from build123d import *

# Parameters (mm, degrees)
SKETCH1_W           = 381
SKETCH1_H           = 508
BOSS_EXTRUDE1_DEPTH = 4.7625
SKETCH2_R           = 14.3383
SKETCH2_R_2         = 2.54
CUT_EXTRUDE1_DEPTH  = 4.7625
SKETCH3_R           = 2.413
CUT_EXTRUDE2_DEPTH  = 4.7625
FILLET1_R           = 2.54


with BuildPart() as part:
    # Sketch1 → Boss-Extrude1 (new body)
    with BuildSketch(Plane(origin=(0, 0, 0), x_dir=(1, 0, 0), z_dir=(0, 1, 0))):
        Rectangle(SKETCH1_W, SKETCH1_H)
    extrude(amount=BOSS_EXTRUDE1_DEPTH)

    # Sketch2 → Cut-Extrude1 (cut)
    with BuildSketch(Plane(origin=(0, 4.7625, 0), x_dir=(1, 0, 0), z_dir=(0, 1, 0))):
        with Locations(Location((-139.7, 228.6, 0), (0, 0, 270))):
            Circle(SKETCH2_R)
        with Locations(Location((-157.660512242, 246.560512242, 0), (0, 0, 270))):
            Circle(SKETCH2_R_2)
        with Locations(Location((-121.739487758, 246.560512242, 0), (0, 0, 270))):
            Circle(SKETCH2_R_2)
        with Locations(Location((-121.739487758, 210.639487758, 0), (0, 0, 270))):
            Circle(SKETCH2_R_2)
        with Locations(Location((-157.660512242, 210.639487758, 0), (0, 0, 270))):
            Circle(SKETCH2_R_2)
        with Locations(Location((-139.7, 177.8, 0), (0, 0, 270))):
            Circle(SKETCH2_R)
        with Locations(Location((-121.739487758, 195.760512242, 0), (0, 0, 270))):
            Circle(SKETCH2_R_2)
        with Locations(Location((-157.660512242, 195.760512242, 0), (0, 0, 270))):
            Circle(SKETCH2_R_2)
        with Locations(Location((-157.660512242, 159.839487758, 0), (0, 0, 270))):
            Circle(SKETCH2_R_2)
        with Locations(Location((-121.739487758, 159.839487758, 0), (0, 0, 270))):
            Circle(SKETCH2_R_2)
        with Locations(Location((-139.7, 127, 0), (0, 0, 270))):
            Circle(SKETCH2_R)
        with Locations(Location((-121.739487758, 144.960512242, 0), (0, 0, 270))):
            Circle(SKETCH2_R_2)
        with Locations(Location((-157.660512242, 144.960512242, 0), (0, 0, 270))):
            Circle(SKETCH2_R_2)
        with Locations(Location((-157.660512242, 109.039487758, 0), (0, 0, 270))):
            Circle(SKETCH2_R_2)
        with Locations(Location((-121.739487758, 109.039487758, 0), (0, 0, 270))):
            Circle(SKETCH2_R_2)
        with Locations(Location((-139.7, 76.2, 0), (0, 0, 270))):
            Circle(SKETCH2_R)
        with Locations(Location((-121.739487758, 94.160512242, 0), (0, 0, 270))):
            Circle(SKETCH2_R_2)
        with Locations(Location((-157.660512242, 94.160512242, 0), (0, 0, 270))):
            Circle(SKETCH2_R_2)
        with Locations(Location((-157.660512242, 58.239487758, 0), (0, 0, 270))):
            Circle(SKETCH2_R_2)
        with Locations(Location((-121.739487758, 58.239487758, 0), (0, 0, 270))):
            Circle(SKETCH2_R_2)
    extrude(amount=-CUT_EXTRUDE1_DEPTH, mode=Mode.SUBTRACT)

    # Sketch3 → Cut-Extrude2 (cut)
    with BuildSketch(Plane(origin=(0, 4.7625, 0), x_dir=(1, 0, 0), z_dir=(0, 1, 0))):
        with Locations(Location((165.1, 228.6, 0), (0, 0, 270))):
            Circle(SKETCH3_R)
        with Locations(Location((165.1, 177.8, 0), (0, 0, 270))):
            Circle(SKETCH3_R)
        with Locations(Location((165.1, 127, 0), (0, 0, 270))):
            Circle(SKETCH3_R)
        with Locations(Location((165.1, 76.2, 0), (0, 0, 270))):
            Circle(SKETCH3_R)
        with Locations(Location((165.1, 25.4, 0), (0, 0, 270))):
            Circle(SKETCH3_R)
        with Locations(Location((165.1, -25.4, 0), (0, 0, 270))):
            Circle(SKETCH3_R)
        with Locations(Location((165.1, -76.2, 0), (0, 0, 270))):
            Circle(SKETCH3_R)
        with Locations(Location((165.1, -127, 0), (0, 0, 270))):
            Circle(SKETCH3_R)
        with Locations(Location((165.1, -177.8, 0), (0, 0, 270))):
            Circle(SKETCH3_R)
        with Locations(Location((165.1, -228.6, 0), (0, 0, 270))):
            Circle(SKETCH3_R)
        with Locations(Location((139.7, 177.8, 0), (0, 0, 270))):
            Circle(SKETCH3_R)
        with Locations(Location((139.7, 127, 0), (0, 0, 270))):
            Circle(SKETCH3_R)
        with Locations(Location((139.7, 76.2, 0), (0, 0, 270))):
            Circle(SKETCH3_R)
        with Locations(Location((139.7, 25.4, 0), (0, 0, 270))):
            Circle(SKETCH3_R)
        with Locations(Location((139.7, -25.4, 0), (0, 0, 270))):
            Circle(SKETCH3_R)
        with Locations(Location((139.7, -76.2, 0), (0, 0, 270))):
            Circle(SKETCH3_R)
        with Locations(Location((139.7, -127, 0), (0, 0, 270))):
            Circle(SKETCH3_R)
        with Locations(Location((139.7, -177.8, 0), (0, 0, 270))):
            Circle(SKETCH3_R)
        with Locations(Location((139.7, -228.6, 0), (0, 0, 270))):
            Circle(SKETCH3_R)
        with Locations(Location((114.3, 177.8, 0), (0, 0, 270))):
            Circle(SKETCH3_R)
        with Locations(Location((114.3, 127, 0), (0, 0, 270))):
            Circle(SKETCH3_R)
        with Locations(Location((114.3, 76.2, 0), (0, 0, 270))):
            Circle(SKETCH3_R)
        with Locations(Location((114.3, 25.4, 0), (0, 0, 270))):
            Circle(SKETCH3_R)
        with Locations(Location((114.3, -25.4, 0), (0, 0, 270))):
            Circle(SKETCH3_R)
        with Locations(Location((114.3, -76.2, 0), (0, 0, 270))):
            Circle(SKETCH3_R)
        with Locations(Location((114.3, -127, 0), (0, 0, 270))):
            Circle(SKETCH3_R)
        with Locations(Location((114.3, -177.8, 0), (0, 0, 270))):
            Circle(SKETCH3_R)
        with Locations(Location((114.3, -228.6, 0), (0, 0, 270))):
            Circle(SKETCH3_R)
        with Locations(Location((139.7, 228.6, 0), (0, 0, 270))):
            Circle(SKETCH3_R)
        with Locations(Location((114.3, 228.6, 0), (0, 0, 270))):
            Circle(SKETCH3_R)
    extrude(amount=-CUT_EXTRUDE2_DEPTH, mode=Mode.SUBTRACT)

    # Fillet1
    fillet1_edges = [part.edges().sort_by_distance(p)[0] for p in [
        (190.5, 2.38125, 254),
        (-190.5, 2.38125, 254),
        (-190.5, 2.38125, -254),
        (190.5, 2.38125, -254),
    ]]
    fillet(fillet1_edges, radius=FILLET1_R)


solid = part.part
Geometry: final body of the model. Coordinates: model frame, mm. Round coordinates to 2 decimals unless told otherwise and drop trailing zeros. Loops run counter-clockwise (first coordinate to the right, second up) from the corner with the lowest first, then second, coordinate; pieces in that order, holes last. Notation, with made-up numbers: M 55.25,23.5 L 97.25,23.5 A25 cw 97.25,45.5 Z; hole C -0.5,12.5 d7. An arc over 180 degrees is marked long. Put each result on its own line as item: value. Start each with the question number.
(1) Draft query along Z for faces 1 (the face through (-3, 4.762, -4)), 2 (the face through (-139.07, 2.415, -242.924)). Return one class per face: +Z half, -Z half, draft (parallel to the pull), parting line (faces both ways), or undercut.
(2) Section query A-A (x = -139.7). Return loops of the section in (y, z), then the cut area to 3 significant figures.
(3) Material intervals for line 1 along X through (y, z) = (1.35, -25.4); line 2 along X through (y, z) = (1.85, -127); line 3 along X through (y, z) = (3.3, -77.5), sorted ascending. Write a range as [from, to].
(4) Contact query for a flat-ended pin moving along its axis: pin 1 Ø4 at (x, z) = (-157.66, -210.64) entering from +Y. Output: stop coordinate, or through.
(5) Section query B-B (y = 3.9). State how many separate pieces and enclosed holes the cut face has, then the cut area to 3 significant figures.
Findings below:
1. face 1: draft
1. face 2: undercut
2. outline: M 0,-254 L 4.76,-254 L 4.76,-242.94 L 0,-242.94 Z; M 0,-214.26 L 4.76,-214.26 L 4.76,-192.14 L 0,-192.14 Z; M 0,-163.46 L 4.76,-163.46 L 4.76,-141.34 L 0,-141.34 Z; M 0,-112.66 L 4.76,-112.66 L 4.76,-90.54 L 0,-90.54 Z; M 0,-61.86 L 4.76,-61.86 L 4.76,254 L 0,254 Z
2. area: 1,870 mm2
3. line 1: x = [-190.5, 111.89], [116.71, 137.29], [142.11, 162.69], [167.51, 190.5]
3. line 2: x = [-190.5, -154.04], [-125.36, 111.89], [116.71, 137.29], [142.11, 162.69], [167.51, 190.5]
3. line 3: x = [-190.5, -153.98], [-125.42, 112.27], [116.33, 137.67], [141.73, 163.07], [167.13, 190.5]
4. pin 1: passes through
5. separate pieces: 1
5. enclosed holes: 50
5. area: 190,000 mm2
